Geometry check sheet. Reference: the model listing, model coordinates, mm. A direction names the side the tool comes from. Round coordinates to 2 decimals unless told otherwise and drop trailing zeros. Loops run counter-clockwise (first coordinate to the right, second up) from the corner with the lowest first, then second, coordinate; pieces in that order, holes last. Notation, with made-up numbers: (32, -25) - (62, -25) arc R27 ccw to (62, -9) - close; hole circle Ø1 at (27.25, 87). An arc over 180 degrees is marked (long way). Write item = value, one per line.
Autodesk Fusion 360 part; units mm, degrees
sketch "Esquisse1" plane through (0, 0, 0) normal (0, 0, 1) x (1, 0, 0)
  line L0 (22.5, 70) -> (57.5, 70)
  line L1 (57.5, 70) -> (57.5, 90)
  line L2 (22.5, 70) -> (22.5, 90)
  line L3 (22.5, 90) -> (12.5, 90)
  line L4 (57.5, 90) -> (67.5, 90)
  line L5 (67.5, 90) -> (67.5, 60)
  line L6 (12.5, 90) -> (12.5, 60)
  line L7 (12.5, 60) -> (25, 5)
  line L8 (25, 5) -> (0, 5)
  line L9 (0, 5) -> (0, 0)
  line L10 (0, 0) -> (80, 0)
  line L11 (80, 0) -> (80, 5)
  line L12 (80, 5) -> (55, 5)
  line L13 (55, 5) -> (67.5, 60)
  dimension "d1" = 70
  dimension "d2" = 35
  dimension "d3" = 20
  dimension "d4" = 10
  dimension "d5" = 30
  dimension "d8" = 5
  dimension "d10" = 10
  dimension "d27" = 80
  dimension "d28" = 55
  dimension "d29" = 12.5
  dimension "d30" = 30
extrude "Extrusion1" add sketch "Esquisse1" along normal blind 90
sketch "Esquisse2" plane through (67.5, 0, 0) normal (1, 0, 0) x (0, 0, -1)
  line L0 (0, 60) -> (0, 90)
  line L1 (0, 90) -> (-90, 90)
  line L2 (-90, 90) -> (-90, 60)
  line L3 (-90, 60) -> (0, 60)
  line L4 (-45, 90) -> (-45, -26) construction
  line L5 (-82, 90) -> (-82, 60)
  line L6 (-82, 60) -> (-60, 5)
  line L7 (-8, 90) -> (-8, 60)
  line L8 (-8, 60) -> (-30, 5)
  line L9 (-60, 5) -> (-30, 5)
  point P0 (-90, 5)
  point P1 (0, 5)
  dimension "d13" = 8
  dimension "d15" = 30
  dimension "d16" = 8
  dimension "d33" = 30
extrude "Extrusion2" cut sketch "Esquisse2" against normal blind 60 contours L3 L6 L8 L9 | L1 L3 L5 L7
sketch "Esquisse3" plane through (0, 0, 90) normal (0, 0, 1) x (1, 0, 0)
  line L0 (22.5, 70) -> (22.5, 90)
  line L1 (22.5, 90) -> (12.5, 90)
  line L2 (12.5, 90) -> (12.5, 60)
  line L3 (12.5, 60) -> (25, 5)
  line L4 (55, 5) -> (67.5, 60)
  line L5 (67.5, 60) -> (67.5, 90)
  line L6 (67.5, 90) -> (57.5, 90)
  line L7 (57.5, 90) -> (57.5, 70)
  line L8 (57.5, 70) -> (22.5, 70)
  line L9 (22.7158, 48.8919) -> (29.534, 18.8919)
  line L10 (34.4097, 15) -> (45.5903, 15)
  line L11 (50.466, 18.8919) -> (57.2842, 48.8919)
  line L12 (52.4085, 55) -> (27.5915, 55)
  arc A0 (27.5915, 55) -> (22.7158, 48.8919) centre (27.5915, 50) ccw
  arc A1 (57.2842, 48.8919) -> (52.4085, 55) centre (52.4085, 50) ccw
  arc A2 (29.534, 18.8919) -> (34.4097, 15) centre (34.4097, 20) ccw
  arc A3 (45.5903, 15) -> (50.466, 18.8919) centre (45.5903, 20) ccw
  line L13 (25, 5) -> (0, 5)
  line L14 (0, 5) -> (0, 0)
  line L15 (0, 0) -> (80, 0)
  line L16 (80, 0) -> (80, 5)
  line L17 (80, 5) -> (55, 5)
  dimension "d20" = 15
  dimension "d21" = 7.5
  dimension "d22" = 7.5
  dimension "d25" = 5
extrude "Extrusion3" cut sketch "Esquisse3" against normal blind 150 contours L9 L10 L11 L12 A0 A1 A2 A3
sketch "Esquisse4" plane through (0, 5, 0) normal (0, 1, 0) x (-1, 0, 0)
  line L0 (-55, 90) -> (-80, 90)
  line L1 (-80, 90) -> (-80, 0)
  line L2 (-80, 0) -> (-55, 0)
  line L3 (-55, 30) -> (-25, 30)
  line L4 (-25, 30) -> (-25, 0)
  line L5 (-25, 0) -> (0, 0)
  line L6 (0, 0) -> (0, 90)
  line L7 (-55, 0) -> (-55, 30)
  line L8 (0, 90) -> (-25, 90)
  circle A0 centre (-40, 45) radius 12.5
  dimension "d34" = 25
extrude "Extrusion4" cut sketch "Esquisse4" against normal blind 20
equation "d15 = d14"
equation "d16 = d13"
equation "d29 = ( d27 - d28 ) / 2"
equation "d33 = d15"
(1) Section check B-B (x = 18). Enter the section's corners in (y, z), then the cut area to 3 significant figures.
Answers follow:
outline = (0, 0) - (5, 0) - (5, 90) - (0, 90) - close; (35.8, 0) - (90, 0) - (90, 8) - (60, 8) - (35.8, 17.68) - close; (35.8, 72.32) - (60, 82) - (90, 82) - (90, 90) - (35.8, 90) - close
area = 1,550 mm²
(2) Set-up check for faces 1 (the flat face through (22.5, 80, 4)), 2 (the flat face through (52.61, 26.77, 21.29)), 3 (the flat face through (40, 55, 5)): record each of +Z, -Z, +X, -X, +Y, -Y from which the full face is reachable in a straight line by a thin tool's end or side.
Answers follow:
face_1 = +Z, -Z, +Y
face_2 = +X, -X, +Y
face_3 = +Z, -Z
(3) Scan lines: L1, parallel to Z at x = 40, y = 1; L2, parallel to Z at x = 60, y = 74; L3, parallel to Y at x = 74, z = 50.5. Record each from-to range of solid material in increasing order. Write a range as [from, to].
Answers follow:
L1 = [0, 32.5], [57.5, 90]
L2 = [0, 8], [82, 90]
L3 = [0, 5]
(4) Mould release check, pull along Y, two halves, no side actions. Record for faces 4 (the flat face through (18, 90, 86)), 5 (the flat face through (57.5, 80, 4)), 6 (the cylindrical face through (23.723, 53.168, 4.926)), 7 (the flat face through (53.827, 33.682, 9.677)): pulls with the +Y half, pulls with the -Y half, needs draft (parallel to the pull), parting line crosses it, or undercut.
Answers follow:
face_4 = pulls with the +Y half
face_5 = needs draft
face_6 = undercut
face_7 = undercut
(5) Section check D-D (y = 74.5). Enter the section's corners in (x, z), then the cut area to 3 significant figures.
Answers follow:
outline = (12.5, 0) - (22.5, 0) - (22.5, 8) - (12.5, 8) - close; (12.5, 82) - (22.5, 82) - (22.5, 90) - (12.5, 90) - close; (57.5, 0) - (67.5, 0) - (67.5, 8) - (57.5, 8) - close; (57.5, 82) - (67.5, 82) - (67.5, 90) - (57.5, 90) - close
area = 320 mm²
(6) Section check A-A (x = 40). Enter the section's corners in (y, z), then the cut area to 4 significant figures.
Answers follow:
outline = (0, 0) - (15, 0) - (15, 26) - (5, 30) - (5, 32.5) - (0, 32.5) - close; (0, 57.5) - (5, 57.5) - (5, 60) - (15, 64) - (15, 90) - (0, 90) - close; (55, 0) - (70, 0) - (70, 8) - (60, 8) - (55, 10) - close; (55, 80) - (60, 82) - (70, 82) - (70, 90) - (55, 90) - close
area = 1,135 mm²
(7) Gauge pin test, flat ends, axial feed: pin 1 (10 mm diameter, centred on y = 37.5, z = 14.5, fed in from -X); pin 2 (4 mm diameter, centred on y = 75.5, z = 85, fed in from -X); pin 3 (8 mm diameter, centred on x = 44.5, z = 86.5, fed in from -Y); pin 4 (9 mm diameter, centred on y = 76.5, z = 5.5, fed in from +X). Record the tip position at first contact, or that the pin passes through.
Answers follow:
pin_1 = 16.48
pin_2 = 12.5
pin_3 = 0
pin_4 = 67.5
(8) Section check C-C (z = 45). Enter the section's corners in (x, y), then the cut area to 3 significant figures.
Answers follow:
outline = (0, 0) - (27.5, 0) - (27.5, 5) - (0, 5) - close; (52.5, 0) - (80, 0) - (80, 5) - (52.5, 5) - close
area = 275 mm²
